from build123d import *

# Parameters (mm, degrees)
IZIM2_W                     = 5
IZIM2_H                     = 6
Y_KSEKLIK_EKSTR_ZYON2_DEPTH = 2


with BuildPart() as part:
    # izim2 → Y_kseklik-Ekstr_zyon2 (new body)
    with BuildSketch(Plane.XY):
        Polygon((24, 0), (0, 7), (0, 0), align=None)
        Polygon((6.48, 11.36), (4.8, 5.6), (12, 3.5), (19.2, 1.4), (20.88, 7.16), align=None)
        with Locations((5.5, -3)):
            Rectangle(IZIM2_W, IZIM2_H)
        with Locations((15.5, -3)):
            Rectangle(IZIM2_W, IZIM2_H)
    extrude(amount=Y_KSEKLIK_EKSTR_ZYON2_DEPTH)


solid = part.part
Read the model definition and answer for the solid it produces. Units are mm, in the model's axes. A direction names the side the tool comes from. Give positions to 0.01 mm unless a question says otherwise; leave off trailing zeros. Loops run counter-clockwise (first coordinate to the right, second up) from the corner with the lowest first, then second, coordinate; pieces in that order, holes last. Notation, with made-up numbers: (26.5, 69.25) - (55.5, 69.25) arc R22 cw to (55.5, 75.25) - close; hole circle Ø9 at (74, 82). An arc over 180 degrees is marked (long way). Answer as CSV lines item,"result". Start each with the question number.
1) Find section D-D (y = 4.25). Write down the section's boundary in (x, z), then the cut area to 3 significant figures.
2) Find section C-C (x = 8.5). Write down the section's boundary in (y, z).
3) Find section A-A (y = -0.5). Write down the section's boundary in (x, z).
4) Which of the six approach directions +Z, -Z, +X, -X, +Y, -Y give full straight-line access (tool end or side, diameter ignored) to faces 5 (the face through (18, -3, 1)), 6 (the face through (1, 0, 1)), 7 (the face through (10, 0, 1)), 8 (the face through (5.65, 8.52, 0.99))?
5) Find section B-B (z = 0.95). Write down the section's boundary in (x, y).
6) Determine the mould class of faces 1 (the face through (2.4, 6.3, 1)), 2 (the face through (21.6, 0.7, 1)), 3 (the face through (3, -3, 1)), 4 (the face through (13, -3, 1)) for opening direction X: released by +X, released by -X, zero draft, split by the parting line, or undercut.
7) Each of these flat-tipped pins is pushed along its axis until it touches: pin 1 Ø0.6 at (y, z) = (-3.5, 1) entering from +X; pin 2 Ø0.6 at (x, z) = (11, 1.5) entering from -Y. Where does it stop, or does it pass through?
8) Straight lines are drawn through the part: L1, parallel to X at y = -2, z = 1.55; L2, parallel to Y at x = 11, z = 1.45; L3, parallel to X at y = 5.5, z = 1.6. For each, find the intervals that lie inside material, in ascending order. Write a range as from..to.
Findings below:
1,outline,"(0, 0) - (20.03, 0) - (20.03, 2) - (0, 2) - close"
1,area,"40.1 mm^2"
2,outline,"(0, 0) - (10.77, 0) - (10.77, 2) - (0, 2) - close"
3,outline,"(3, 0) - (8, 0) - (8, 2) - (3, 2) - close; (13, 0) - (18, 0) - (18, 2) - (13, 2) - close"
4,face 5,"+Z, -Z, +X, -Y"
4,face 6,"+Z, -Z, -X, -Y"
4,face 7,"+Z, -Z, -Y"
4,face 8,"+Z, -Z, +Y"
5,outline,"(0, 0) - (3, 0) - (3, -6) - (8, -6) - (8, 0) - (13, 0) - (13, -6) - (18, -6) - (18, 0) - (24, 0) - (19.2, 1.4) - (20.88, 7.16) - (6.48, 11.36) - (4.8, 5.6) - (0, 7) - close"
6,face 1,"undercut"
6,face 2,"released by +X"
6,face 3,"released by -X"
6,face 4,"undercut"
7,pin 1,"x = 18"
7,pin 2,"y = 0"
8,L1,"3..8, 13..18"
8,L2,"0..10.04"
8,L3,"0..20.4"
